```python
from build123d import *

# Parameters (mm, degrees)
SKETCH_1_W          = 8
SKETCH_1_H          = 8
EXTRUDE_1_DEPTH     = 10
SKETCH_4_R          = 2.5
CUT_EXTRUDE_2_DEPTH = 9
FILLET_1_R          = 1


with BuildPart() as part:
    # 草图1 → 凸台-拉伸1 (new body)
    with BuildSketch(Plane.XY):
        with Locations((4, 4)):
            Rectangle(SKETCH_1_W, SKETCH_1_H)
    extrude(amount=EXTRUDE_1_DEPTH)

    # 草图4 → 切除-拉伸2 (cut, through all)
    with BuildSketch(Plane(origin=(8, 0, 0), x_dir=(0, 0, -1), z_dir=(1, 0, 0))):
        with Locations((-5, 4)):
            Circle(SKETCH_4_R)
    extrude(amount=-CUT_EXTRUDE_2_DEPTH, mode=Mode.SUBTRACT)

    # 圆角1
    fillet_1_edges = [part.edges().sort_by_distance(p)[0] for p in [
        (8, 4, 10),
        (4, 8, 10),
        (0, 4, 10),
        (4, 8, 0),
        (8, 4, 0),
        (4, 0, 0),
        (0, 4, 0),
        (0, 8, 5),
        (8, 8, 5),
        (8, 0, 5),
        (0, 0, 5),
        (4, 0, 10),
    ]]
    fillet(fillet_1_edges, radius=FILLET_1_R)


solid = part.part
```
Here's how the part is built. I have some questions about the finished solid (model axes, mm). Give positions to 0.01 mm unless a question says otherwise; leave off trailing zeros. Write each loop counter-clockwise with the first axis right and the second up, starting at its lowest first coordinate (ties: lowest second). Pieces come first, ordered by that corner, then holes. Notation, with made-up numbers: M 64,-12 L 121,-12 A12 cw 121,-7 Z; hole C -28,0 d1. An arc over 180 degrees is marked long. Put each result on its own line as item: value. Start each with the question number.
Item 1: I need wall thicknesses on L1, parallel to Y at x = 6.25, z = 5; L2, parallel to Z at x = 1.5, y = 5.5; L3, parallel to Y at x = 3, z = 3.5. Which ranges of each line are inside material? Lowest first, please. Write a range as from..to.
Item 2: If we section it at A-A, the plane y = 4: Write out the boundary of the cut face in (x, z), then the cut area to 3 significant figures.
Item 3: If we section it at B-B, the plane x = 3.25: Write out the boundary of the cut face in (y, z).
Item 4: If we section it at D-D, the plane y = 7.25: Write out the boundary of the cut face in (x, z), then the cut area to 3 significant figures.
Item 5: If we section it at C-C, the plane z = 5: Write out the boundary of the cut face in (x, y), then the cut area to 3 significant figures.
Values:
1. L1: 0..1.5, 6.5..8
1. L2: 0..3, 7..10
1. L3: 0..2, 6..8
2. outline: M 0,1 A1 ccw 1,0 L 7,0 A1 ccw 8,1 L 8,2.5 L 0,2.5 Z; M 0,7.5 L 8,7.5 L 8,9 A1 ccw 7,10 L 1,10 A1 ccw 0,9 Z
2. area: 39.1 mm²
3. outline: M 0,1 A1 ccw 1,0 L 7,0 A1 ccw 8,1 L 8,9 A1 ccw 7,10 L 1,10 A1 ccw 0,9 Z; hole C 4,5 d5
4. outline: M 0.03,1 A0.97 ccw 1,0.03 L 7,0.03 A0.97 ccw 7.97,1 L 7.97,9 A0.97 ccw 7,9.97 L 1,9.97 A0.97 ccw 0.03,9 Z
4. area: 78.1 mm²
5. outline: M 0,1 A1 ccw 1,0 L 7,0 A1 ccw 8,1 L 8,1.5 L 0,1.5 Z; M 0,6.5 L 8,6.5 L 8,7 A1 ccw 7,8 L 1,8 A1 ccw 0,7 Z
5. area: 23.1 mm²
